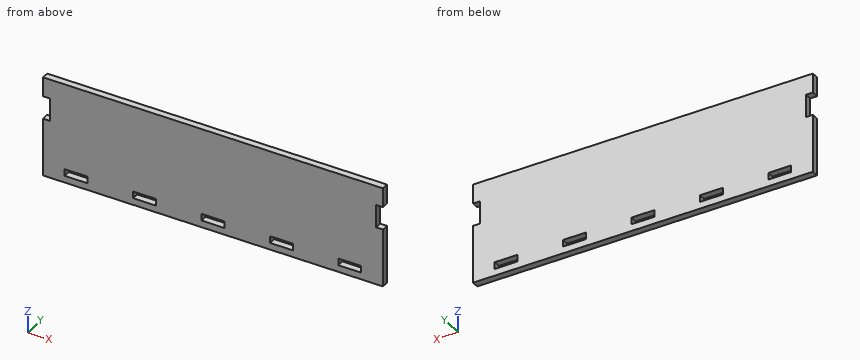
```python
from build123d import *

# Parameters (mm, degrees)
SKETCH1_W           = 10
SKETCH1_H           = 3
BOSS_EXTRUDE1_DEPTH = 3


with BuildPart() as part:
    # Sketch1 → Boss-Extrude1 (new body)
    with BuildSketch(Plane(origin=(0, 0, 0), x_dir=(1, 0, 0), z_dir=(0, 1, 0))):
        Polygon((-74.5, 44), (74.5, 44), (74.5, 18.5), (71.5, 18.5), (71.5, 8.5), (74.5, 8.5), (74.5, 0), (-74.5, 0), (-74.5, 8.5), (-71.5, 8.5), (-71.5, 18.5), (-74.5, 18.5), align=None)
        with Locations((0, 39.5)):
            Rectangle(SKETCH1_W, SKETCH1_H, mode=Mode.SUBTRACT)
        with Locations((30, 39.5)):
            Rectangle(SKETCH1_W, SKETCH1_H, mode=Mode.SUBTRACT)
        with Locations((60, 39.5)):
            Rectangle(SKETCH1_W, SKETCH1_H, mode=Mode.SUBTRACT)
        with Locations((-60, 39.5)):
            Rectangle(SKETCH1_W, SKETCH1_H, mode=Mode.SUBTRACT)
        with Locations((-30, 39.5)):
            Rectangle(SKETCH1_W, SKETCH1_H, mode=Mode.SUBTRACT)
    extrude(amount=BOSS_EXTRUDE1_DEPTH)


solid = part.part
```
Check sheet for the modelled part. Datum: model origin and axes. Units: mm. Give positions to 0.01 mm unless a question says otherwise; leave off trailing zeros. Write each loop counter-clockwise with the first axis right and the second up, starting at its lowest first coordinate (ties: lowest second). Pieces come first, ordered by that corner, then holes.
Item 1: Gauge pin test, flat ends, axial feed: pin 1 (1 mm diameter, centred on y = 2.5, z = -11.5, fed in from +X); pin 2 (10 mm diameter, centred on x = 25.5, z = -21.5, fed in from -Y); pin 3 (0.9 mm diameter, centred on y = 2, z = -11, fed in from -X). Record the tip position at first contact, or that the pin passes through.
Item 2: Cross-section at A-A (x = -1.5). Enter the section's corners in (y, z).
Item 3: Scan lines: L1, parallel to Z at x = -60, y = 2.2; L2, parallel to X at y = 1.85, z = -39; L3, parallel to X at y = 0.9, z = -17. Record each from-to range of solid material in increasing order.
Item 4: Cross-section at B-B (y = 1.95). Count the separate pieces of the cut face and the enclosed holes in it, and give its area (3 significant figures).
Report:
1. pin 1: stops at x = 71.5
1. pin 2: stops at y = 0
1. pin 3: stops at x = -71.5
2. outline: (0, -44) - (3, -44) - (3, -41) - (0, -41) - close; (0, -38) - (3, -38) - (3, 0) - (0, 0) - close
3. L1: z = -44 to -41, -38 to 0
3. L2: x = -74.5 to -65, -55 to -35, -25 to -5, 5 to 25, 35 to 55, 65 to 74.5
3. L3: x = -71.5 to 71.5
4. separate pieces: 1
4. enclosed holes: 5
4. area: 6,350 mm2
